```python
from build123d import *

# Parameters (mm, degrees)
SALIENTE_EXTRUIR1_DEPTH = 196
CORTAR_EXTRUIR1_REACH   = 266.89
CROQUIS2_W              = 37.5
CROQUIS2_H              = 62.989872981
CORTAR_EXTRUIR2_REACH   = 266.89
CROQUIS4_W              = 13
CROQUIS4_H              = 22.5
CUT_EXTRUDE1_REACH      = 266.89
SKETCH1_R               = 1.585
CUT_EXTRUDE2_REACH      = 266.89
SKETCH2_R               = 1.585
CUT_EXTRUDE3_REACH      = 266.89
SKETCH3_R               = 1.585
SKETCH4_R               = 2.5
SKETCH4_R_2             = 1.6
BOSS_EXTRUDE1_DEPTH     = 5
SKETCH8_R               = 1.6
CUT_EXTRUDE6_DEPTH      = 265.925553505
FILLET1_R               = 3
SKETCH12_R              = 1.575419973
CUT_EXTRUDE9_DEPTH      = 10
SKETCH14_R              = 1.575419973
CUT_EXTRUDE10_DEPTH     = 10


with BuildPart() as part:
    # Croquis1 → Saliente-Extruir1 (new body)
    with BuildSketch(Plane(origin=(0, 0, 0), x_dir=(0, 0, -1), z_dir=(1, 0, 0))):
        Polygon((0, 0), (178.17, 0), (178.17, 2.5), (9.330127019, 2.5), align=None)
    extrude(amount=SALIENTE_EXTRUIR1_DEPTH)

    # Croquis2 → Cortar-Extruir1 (cut, up to next)
    with BuildSketch(Plane(origin=(0, 0, 0), x_dir=(-1, 0, 0), z_dir=(0, -1, 0)), mode=Mode.PRIVATE) as cortar_extruir1_sk1:
        with Locations((-18.75, 146.67506351)):
            Rectangle(CROQUIS2_W, CROQUIS2_H)
    cortar_extruir1_tool1 = extrude(cortar_extruir1_sk1.sketch, amount=-CORTAR_EXTRUIR1_REACH, mode=Mode.PRIVATE) & part.part
    # Croquis2 → Cortar-Extruir1 (cut, up to next)
    with BuildSketch(Plane(origin=(0, 0, 0), x_dir=(-1, 0, 0), z_dir=(0, -1, 0)), mode=Mode.PRIVATE) as cortar_extruir1_sk2:
        with Locations((-177.25, 146.67506351)):
            Rectangle(CROQUIS2_W, CROQUIS2_H)
    cortar_extruir1_tool2 = extrude(cortar_extruir1_sk2.sketch, amount=-CORTAR_EXTRUIR1_REACH, mode=Mode.PRIVATE) & part.part
    add(cortar_extruir1_tool1.solids().sort_by_distance((18.75, 0, -146.675064))[0], mode=Mode.SUBTRACT)
    add(cortar_extruir1_tool2.solids().sort_by_distance((177.25, 0, -146.675064))[0], mode=Mode.SUBTRACT)

    # Croquis4 → Cortar-Extruir2 (cut, up to next)
    with BuildSketch(Plane(origin=(0, 2.5, 0), x_dir=(1, 0, 0), z_dir=(0, 1, 0)), mode=Mode.PRIVATE) as cortar_extruir2_sk1:
        with Locations((10.5, 24.580127019)):
            Rectangle(CROQUIS4_W, CROQUIS4_H)
    cortar_extruir2_tool1 = extrude(cortar_extruir2_sk1.sketch, amount=-CORTAR_EXTRUIR2_REACH, mode=Mode.PRIVATE) & part.part
    cortar_extruir2 = cortar_extruir2_tool1.solids().sort_by_distance((10.5, 2.5, -24.580127))[0]
    add(cortar_extruir2, mode=Mode.SUBTRACT)

    # Simetría1: Cortar-Extruir2 across plane
    add(cortar_extruir2.mirror(Plane(origin=(98, 0, 0), x_dir=(0, 0, 1), z_dir=(1, 0, 0))), mode=Mode.SUBTRACT)

    # Sketch1 → Cut-Extrude1 (cut, up to next)
    with BuildSketch(Plane(origin=(0, 2.5, 0), x_dir=(1, 0, 0), z_dir=(0, 1, 0)), mode=Mode.PRIVATE) as cut_extrude1_sk1:
        with Locations(Location((187.5, 106.180127019, 0), (0, 0, 270))):
            Circle(SKETCH1_R)
    cut_extrude1_tool1 = extrude(cut_extrude1_sk1.sketch, amount=-CUT_EXTRUDE1_REACH, mode=Mode.PRIVATE) & part.part
    # Sketch1 → Cut-Extrude1 (cut, up to next)
    with BuildSketch(Plane(origin=(0, 2.5, 0), x_dir=(1, 0, 0), z_dir=(0, 1, 0)), mode=Mode.PRIVATE) as cut_extrude1_sk2:
        with Locations(Location((8.5, 106.180127019, 0), (0, 0, 270))):
            Circle(SKETCH1_R)
    cut_extrude1_tool2 = extrude(cut_extrude1_sk2.sketch, amount=-CUT_EXTRUDE1_REACH, mode=Mode.PRIVATE) & part.part
    add(cut_extrude1_tool1.solids().sort_by_distance((187.5, 2.5, -106.180127))[0], mode=Mode.SUBTRACT)
    add(cut_extrude1_tool2.solids().sort_by_distance((8.5, 2.5, -106.180127))[0], mode=Mode.SUBTRACT)

    # Sketch2 → Cut-Extrude2 (cut, up to next)
    with BuildSketch(Plane(origin=(0, 2.5, 0), x_dir=(1, 0, 0), z_dir=(0, 1, 0)), mode=Mode.PRIVATE) as cut_extrude2_sk1:
        with Locations(Location((98.5, 26.180127019, 0), (0, 0, 270))):
            Circle(SKETCH2_R)
    cut_extrude2_tool1 = extrude(cut_extrude2_sk1.sketch, amount=-CUT_EXTRUDE2_REACH, mode=Mode.PRIVATE) & part.part
    add(cut_extrude2_tool1.solids().sort_by_distance((98.5, 2.5, -26.180127))[0], mode=Mode.SUBTRACT)

    # Sketch3 → Cut-Extrude3 (cut, up to next)
    with BuildSketch(Plane(origin=(0, 2.5, 0), x_dir=(1, 0, 0), z_dir=(0, 1, 0)), mode=Mode.PRIVATE) as cut_extrude3_sk1:
        with Locations(Location((111.5, 124.67, 0), (0, 0, 270))):
            Circle(SKETCH3_R)
    cut_extrude3_tool1 = extrude(cut_extrude3_sk1.sketch, amount=-CUT_EXTRUDE3_REACH, mode=Mode.PRIVATE) & part.part
    # Sketch3 → Cut-Extrude3 (cut, up to next)
    with BuildSketch(Plane(origin=(0, 2.5, 0), x_dir=(1, 0, 0), z_dir=(0, 1, 0)), mode=Mode.PRIVATE) as cut_extrude3_sk2:
        with Locations(Location((152.5, 124.67, 0), (0, 0, 270))):
            Circle(SKETCH3_R)
    cut_extrude3_tool2 = extrude(cut_extrude3_sk2.sketch, amount=-CUT_EXTRUDE3_REACH, mode=Mode.PRIVATE) & part.part
    # Sketch3 → Cut-Extrude3 (cut, up to next)
    with BuildSketch(Plane(origin=(0, 2.5, 0), x_dir=(1, 0, 0), z_dir=(0, 1, 0)), mode=Mode.PRIVATE) as cut_extrude3_sk3:
        with Locations(Location((152.5, 173.17, 0), (0, 0, 270))):
            Circle(SKETCH3_R)
    cut_extrude3_tool3 = extrude(cut_extrude3_sk3.sketch, amount=-CUT_EXTRUDE3_REACH, mode=Mode.PRIVATE) & part.part
    # Sketch3 → Cut-Extrude3 (cut, up to next)
    with BuildSketch(Plane(origin=(0, 2.5, 0), x_dir=(1, 0, 0), z_dir=(0, 1, 0)), mode=Mode.PRIVATE) as cut_extrude3_sk4:
        with Locations(Location((111.5, 173.17, 0), (0, 0, 270))):
            Circle(SKETCH3_R)
    cut_extrude3_tool4 = extrude(cut_extrude3_sk4.sketch, amount=-CUT_EXTRUDE3_REACH, mode=Mode.PRIVATE) & part.part
    # Sketch3 → Cut-Extrude3 (cut, up to next)
    with BuildSketch(Plane(origin=(0, 2.5, 0), x_dir=(1, 0, 0), z_dir=(0, 1, 0)), mode=Mode.PRIVATE) as cut_extrude3_sk5:
        with Locations(Location((84.5, 173.17, 0), (0, 0, 270))):
            Circle(SKETCH3_R)
    cut_extrude3_tool5 = extrude(cut_extrude3_sk5.sketch, amount=-CUT_EXTRUDE3_REACH, mode=Mode.PRIVATE) & part.part
    # Sketch3 → Cut-Extrude3 (cut, up to next)
    with BuildSketch(Plane(origin=(0, 2.5, 0), x_dir=(1, 0, 0), z_dir=(0, 1, 0)), mode=Mode.PRIVATE) as cut_extrude3_sk6:
        with Locations(Location((43.5, 173.17, 0), (0, 0, 270))):
            Circle(SKETCH3_R)
    cut_extrude3_tool6 = extrude(cut_extrude3_sk6.sketch, amount=-CUT_EXTRUDE3_REACH, mode=Mode.PRIVATE) & part.part
    # Sketch3 → Cut-Extrude3 (cut, up to next)
    with BuildSketch(Plane(origin=(0, 2.5, 0), x_dir=(1, 0, 0), z_dir=(0, 1, 0)), mode=Mode.PRIVATE) as cut_extrude3_sk7:
        with Locations(Location((43.5, 124.67, 0), (0, 0, 270))):
            Circle(SKETCH3_R)
    cut_extrude3_tool7 = extrude(cut_extrude3_sk7.sketch, amount=-CUT_EXTRUDE3_REACH, mode=Mode.PRIVATE) & part.part
    # Sketch3 → Cut-Extrude3 (cut, up to next)
    with BuildSketch(Plane(origin=(0, 2.5, 0), x_dir=(1, 0, 0), z_dir=(0, 1, 0)), mode=Mode.PRIVATE) as cut_extrude3_sk8:
        with Locations(Location((84.5, 124.67, 0), (0, 0, 270))):
            Circle(SKETCH3_R)
    cut_extrude3_tool8 = extrude(cut_extrude3_sk8.sketch, amount=-CUT_EXTRUDE3_REACH, mode=Mode.PRIVATE) & part.part
    add(cut_extrude3_tool1.solids().sort_by_distance((111.5, 2.5, -124.67))[0], mode=Mode.SUBTRACT)
    add(cut_extrude3_tool2.solids().sort_by_distance((152.5, 2.5, -124.67))[0], mode=Mode.SUBTRACT)
    add(cut_extrude3_tool3.solids().sort_by_distance((152.5, 2.5, -173.17))[0], mode=Mode.SUBTRACT)
    add(cut_extrude3_tool4.solids().sort_by_distance((111.5, 2.5, -173.17))[0], mode=Mode.SUBTRACT)
    add(cut_extrude3_tool5.solids().sort_by_distance((84.5, 2.5, -173.17))[0], mode=Mode.SUBTRACT)
    add(cut_extrude3_tool6.solids().sort_by_distance((43.5, 2.5, -173.17))[0], mode=Mode.SUBTRACT)
    add(cut_extrude3_tool7.solids().sort_by_distance((43.5, 2.5, -124.67))[0], mode=Mode.SUBTRACT)
    add(cut_extrude3_tool8.solids().sort_by_distance((84.5, 2.5, -124.67))[0], mode=Mode.SUBTRACT)

    # Sketch4 → Boss-Extrude1 (add)
    # profile 1 of 2: a face of its own
    with BuildSketch(Plane(origin=(0, 2.5, 0), x_dir=(1, 0, 0), z_dir=(0, 1, 0))):
        with Locations(Location((68.415265875, 108.280438226, 0), (0, 0, 90))):
            Circle(SKETCH4_R)
        with Locations(Location((68.415265875, 108.280438226, 0), (0, 0, 270))):
            Circle(SKETCH4_R_2, mode=Mode.SUBTRACT)
    # profile 2 of 2: a face of its own
    with BuildSketch(Plane(origin=(0, 2.5, 0), x_dir=(1, 0, 0), z_dir=(0, 1, 0))):
        with Locations(Location((125.876416732, 108.336862559, 0), (0, 0, 90))):
            Circle(SKETCH4_R)
        with Locations(Location((125.876416732, 108.336862559, 0), (0, 0, 270))):
            Circle(SKETCH4_R_2, mode=Mode.SUBTRACT)
    extrude(amount=BOSS_EXTRUDE1_DEPTH)

    # Sketch8 → Cut-Extrude6 (cut, through all)
    with BuildSketch(Plane(origin=(0, 2.5, 0), x_dir=(1, 0, 0), z_dir=(0, 1, 0))):
        with Locations(Location((68.415265875, 108.280438226, 0), (0, 0, 270))):
            Circle(SKETCH8_R)
        with Locations(Location((125.876416732, 108.336862559, 0), (0, 0, 270))):
            Circle(SKETCH8_R)
    extrude(amount=-CUT_EXTRUDE6_DEPTH, mode=Mode.SUBTRACT)

    # Fillet1
    fillet1_edges = [part.edges().sort_by_distance(p)[0] for p in [
        (68.415265875, 2.5, -105.780438226),
        (125.876416732, 2.5, -105.836862559),
    ]]
    fillet(fillet1_edges, radius=FILLET1_R)

    # Sketch12 → Cut-Extrude9 (cut)
    with BuildSketch(Plane(origin=(0, 2.5, 0), x_dir=(1, 0, 0), z_dir=(0, 1, 0))):
        with Locations(Location((20.010826356, 47.41770363, 0), (0, 0, 270))):
            Circle(SKETCH12_R)
        with Locations(Location((63.468062002, 35.773372434, 0), (0, 0, 270))):
            Circle(SKETCH12_R)
        with Locations(Location((129.523650189, 34.779634544, 0), (0, 0, 270))):
            Circle(SKETCH12_R)
        with Locations(Location((173.36079416, 44.900236676, 0), (0, 0, 270))):
            Circle(SKETCH12_R)
    extrude(amount=-CUT_EXTRUDE9_DEPTH, mode=Mode.SUBTRACT)

    # Sketch14 → Cut-Extrude10 (cut)
    with BuildSketch(Plane(origin=(0, 2.5, 0), x_dir=(1, 0, 0), z_dir=(0, 1, 0))):
        with Locations(Location((76.242264521, 68.095650208, 0), (0, 0, 270))):
            Circle(SKETCH14_R)
        with Locations(Location((121.232505451, 68.095650208, 0), (0, 0, 270))):
            Circle(SKETCH14_R)
    extrude(amount=-CUT_EXTRUDE10_DEPTH, mode=Mode.SUBTRACT)


solid = part.part
```
Verification items for the finished model (mm, model axes). Give positions to 0.01 mm unless a question says otherwise; leave off trailing zeros. Order: outer loops, then holes, each group sorted by start corner. A loop starts at its lowest first (then second) coordinate and runs counter-clockwise, first axis right, second up. Notation, with made-up numbers: (38, -33.5) -> (88, -33.5) arc R34 ccw to (88, 2.5) -> close; hole circle Ø6 at (23, -12.5). An arc over 180 degrees is marked (long way). One line per item, written item: value.
(1) Scan lines: line 1 along X through (y, z) = (0.95, -124.67) (3 decimals); line 2 along Y through (x, z) = (101.5, -105). Record each from-to range of solid material in increasing order. Write a range as [from, to].
Final values:
line 1: [37.5, 41.915], [45.085, 82.915], [86.085, 109.915], [113.085, 150.915], [154.085, 158.5]
line 2: [0, 2.5]
(2) Sectioned sample at A-A on x = 13. Record the cut outline in (y, z).
Final values:
outline: (0, -115.18) -> (2.5, -115.18) -> (2.5, -35.83) -> (0, -35.83) -> close; (0, -13.33) -> (2.5, -13.33) -> (2.5, -9.33) -> (0, 0) -> close
(3) Sectioned sample at C-C on x = 104.5. Record the cut outline in (y, z).
Final values:
outline: (0, -178.17) -> (2.5, -178.17) -> (2.5, -9.33) -> (0, 0) -> close
(4) Draft check along X on faces 1 (the face through (127.398, 6.486, -106.353)), 2 (the face through (96.628, 1.267, -4.73)), 3 (the face through (68.305, 6.486, -105.783)). Enter one of: pulls with the +X half, pulls with the -X half, needs draft (parallel to the pull), parting line crosses it, or undercut.
Final values:
face 1: undercut
face 2: needs draft
face 3: undercut
(5) Sectioned sample at B-B on z = -97. Record the cut outline in (x, y), then the cut area to 3 significant figures.
Final values:
outline: (0, 0) -> (196, 0) -> (196, 2.5) -> (0, 2.5) -> close
area: 490 mm^2
(6) Gauge pin test, flat ends, axial feed: pin 1 (5 mm diameter, centred on x = 173.36, z = -44.9, fed in from +Y); pin 2 (3.5 mm diameter, centred on x = 111.5, z = -173.17, fed in from -Y); pin 3 (1.2 mm diameter, centred on y = 1, z = -143.5, fed in from +X); pin 4 (2 mm diameter, centred on x = 186.5, y = 0.5, fed in from -Z). Record the tip position at first contact, or that the pin passes through.
Final values:
pin 1: y = 2.5
pin 2: y = 0
pin 3: x = 158.5
pin 4: z = -115.18
